Verification items for the finished model (mm, model axes). Round coordinates to 2 decimals unless told otherwise and drop trailing zeros. Order: outer loops, then holes, each group sorted by start corner. A loop starts at its lowest first (then second) coordinate and runs counter-clockwise, first axis right, second up. Notation, with made-up numbers: (81, 67) -> (131, 67) arc R8 ccw to (131, 81) -> close; hole circle Ø7 at (81, 77.25). An arc over 180 degrees is marked (long way). Return JSON: item names as keys, results as strings. Group by question number.
1) Depth check by flat-ended pin: pin 1 (10 mm diameter, centred on x = 10, y = 28.5, fed in from -Z). Enter the tip coordinate at first touch or a pass-through.
2) Section check B-B on z = 433.5. Enter the section's corners in (x, y) (3 decimals), plus the area to 3 significant figures.
3) Scan lines: L1, parallel to Y at x = 2.25, z = 12.7; L2, parallel to X at y = 46.5, z = 366 (3 decimals); L3, parallel to Y at x = 13.5, z = 450.5 (3 decimals). Record each from-to range of solid material in increasing order.
4) Section check A-A on y = 28. Enter the section's corners in (x, z) (3 decimals), plus the area to 3 significant figures.
5) Section check C-C on x = 18. Enter the section's corners in (y, z) (3 decimals).
Autodesk Inventor part; units mm, degrees
ref_plane "YZ Plane" through (0, 0, 0) normal (1, 0, 0) x (0, 1, 0)
ref_plane "XZ Plane" through (0, 0, 0) normal (0, 1, 0) x (-1, 0, 0)
ref_plane "XY Plane" through (0, 0, 0) normal (0, 0, 1) x (1, 0, 0)
sketch "Sketch1" plane through (0, 0, 0) normal (0, 0, 1) x (1, 0, 0)
  line L0 (0, 0) -> (25.4, 0)
  line L1 (25.4, 0) -> (25.4, 50.8)
  line L2 (25.4, 50.8) -> (0, 50.8)
  line L3 (0, 50.8) -> (0, 0)
  line L4 (22.225, 47.625) -> (22.225, 3.175)
  line L5 (22.225, 3.175) -> (3.175, 3.175)
  line L6 (3.175, 3.175) -> (3.175, 47.625)
  line L7 (3.175, 47.625) -> (22.225, 47.625)
  dimension "d0" = 25.4
  dimension "d1" = 50.8
  dimension "d2" = 3.175
extrude "Extrusion1" add sketch "Sketch1" along normal blind 762
sketch "Sketch2" plane through (25.4, 0, 0) normal (1, 0, 0) x (0, 0, -1)
  line L0 (0, 0) -> (-12.7, 0)
  line L1 (0, 0) -> (-762, 0)
  line L2 (-12.7, 0) -> (-12.7, 50.8)
  line L3 (0, 50.8) -> (-762, 50.8)
  line L4 (-12.7, 50.8) -> (-38.1, 50.8)
  line L5 (-38.1, 50.8) -> (-38.1, 0)
  line L6 (-12.7, 50.8) -> (-12.7, 38.1)
  line L7 (-12.7, 38.1) -> (-38.1, 38.1)
  line L8 (-38.1, 0) -> (-38.1, 12.7)
  line L9 (-38.1, 12.7) -> (-12.7, 12.7)
  circle A0 centre (-38.1, 38.1) radius 2.54
  circle A1 centre (-12.7, 38.1) radius 2.54
  circle A2 centre (-12.7, 12.7) radius 2.54
  circle A3 centre (-38.1, 12.7) radius 2.54
  line L10 (-381, 50.8) -> (-381, 0)
  line L11 (-762, 0) -> (-749.3, 0)
  line L12 (-762, 0) -> (0, 0)
  line L13 (-749.3, 0) -> (-749.3, 50.8)
  line L14 (-762, 50.8) -> (0, 50.8)
  line L15 (-749.3, 50.8) -> (-723.9, 50.8)
  line L16 (-723.9, 50.8) -> (-723.9, 0)
  line L17 (-749.3, 50.8) -> (-749.3, 38.1)
  line L18 (-749.3, 38.1) -> (-723.9, 38.1)
  line L19 (-723.9, 0) -> (-723.9, 12.7)
  line L20 (-723.9, 12.7) -> (-749.3, 12.7)
  circle A4 centre (-723.9, 38.1) radius 2.54
  circle A5 centre (-749.3, 38.1) radius 2.54
  circle A6 centre (-749.3, 12.7) radius 2.54
  circle A7 centre (-723.9, 12.7) radius 2.54
  dimension "d5" = 12.7
  dimension "d6" = 25.4
  dimension "d7" = 12.7
  dimension "d8" = 12.7
  dimension "d9" = 5.08
  dimension "d10" = 5.08
  dimension "d11" = 5.08
  dimension "d12" = 5.08
extrude "Extrusion2" cut sketch "Sketch2" against normal blind 762 contours A2 L9 L2 | L2 A2 | A3 L5 | L5 L9 A3 | L9 A2 L2 | L5 A3 L9 | A7 L20 L16 | L16 A7 | A0 L5 | L5 L7 A0 | A1 L7 L2 | L2 A1 | A6 L13 | L13 L20 A6 | L20 A7 L16 | A0 L7 L5 | A4 L16 | L16 L18 A4 | L7 A1 L2 | L13 A6 L20 | A5 L18 L13 | L13 A5 | L16 A4 L18 | L13 L18 A5
sketch "Sketch3" plane through (25.4, 0, 0) normal (1, 0, 0) x (0, 0, -1)
  line L0 (0, 0) -> (-114.3, 0)
  line L1 (0, 0) -> (-762, 0)
  line L2 (-114.3, 0) -> (-114.3, 50.8)
  line L3 (0, 50.8) -> (-762, 50.8)
  circle A0 centre (-114.3, 38.1) radius 2.54
  circle A1 centre (-114.3, 12.7) radius 2.54
  line L4 (0, 47.625) -> (-762, 47.625)
  line L5 (-381, 47.625) -> (-381, 0)
  circle A2 centre (-647.7, 38.1) radius 2.54
  circle A3 centre (-647.7, 12.7) radius 2.54
  circle A4 centre (-381, 38.1) radius 2.54
  circle A5 centre (-381, 12.7) radius 2.54
  dimension "d15" = 114.3
  dimension "d16" = 5.08
extrude "Extrusion3" cut sketch "Sketch3" against normal blind 25.4 contours A1 L2 | L2 A1 | A5 L5 | L5 A5 | A0 L2 | L2 A0 | A4 L5 | L5 A4 | A2 | A3
properties part number "1x2x30"
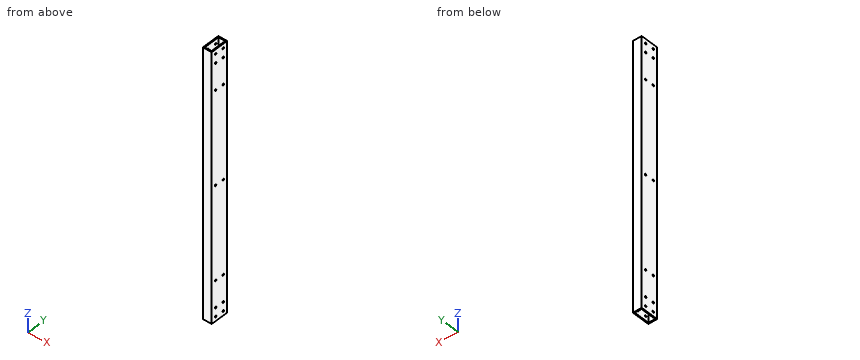
Check result:
{
 "1": {"pin 1": "through"},
 "2": {"outline": "(0, 0) -> (25.4, 0) -> (25.4, 50.8) -> (0, 50.8) -> close; hole (3.175, 3.175) -> (22.225, 3.175) -> (22.225, 47.625) -> (3.175, 47.625) -> close", "area": "444 mm^2"},
 "3": {"L1": "0 to 10.16, 15.24 to 35.56, 40.64 to 50.8", "L2": "0 to 3.175, 22.225 to 25.4", "L3": "0 to 3.175, 47.625 to 50.8"},
 "4": {"outline": "(0, 0) -> (3.175, 0) -> (3.175, 762) -> (0, 762) -> close; (22.225, 0) -> (25.4, 0) -> (25.4, 762) -> (22.225, 762) -> close", "area": "4,840 mm^2"},
 "5": {"outline": "(0, 0) -> (3.175, 0) -> (3.175, 762) -> (0, 762) -> close; (47.625, 0) -> (50.8, 0) -> (50.8, 762) -> (47.625, 762) -> close"}
}
